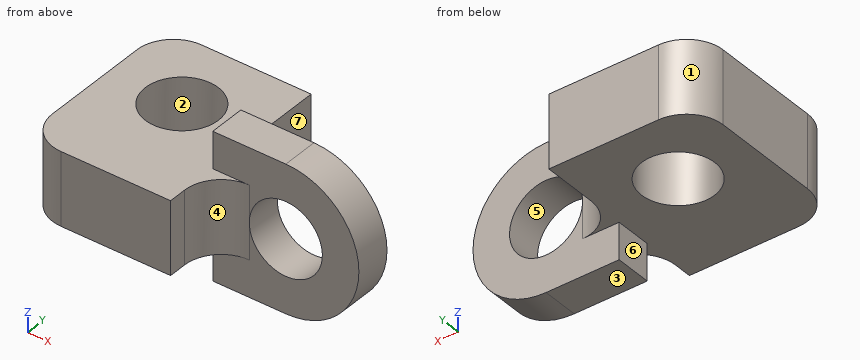
```python
from build123d import *

# Parameters (mm, degrees)
SKETCH_1_R      = 5
EXTRUDE_1_DEPTH = 2.5
SKETCH_2_R      = 5
EXTRUDE_2_DEPTH = 5
FILLET_1_R      = 5
SCALE_1_SCALE   = 0.2


with BuildPart() as part:
    # 草圖1 → 填料-伸長1 (new, symmetric)
    with BuildSketch(Plane(origin=(0, 0, 0), x_dir=(1, 0, 0), z_dir=(0, 1, 0))):
        with BuildLine():
            Line((0, 10), (-10, 10))
            Line((-10, 10), (-10, -10))
            Line((-10, -10), (0, -10))
            ThreePointArc((0, -10), (10, 0), (0, 10))
        make_face()
        with Locations(Location((0, 0, 0), (0, 0, 270))):
            Circle(SKETCH_1_R, mode=Mode.SUBTRACT)
    extrude(amount=EXTRUDE_1_DEPTH, both=True)

    # 草圖2 → 填料-伸長2 (add, symmetric)
    with BuildSketch(Plane.XY):
        with BuildLine():
            Line((-30, 1.898257061), (-30, -5))
            ThreePointArc((-30, -5), (-28.535533906, -8.535533906), (-25, -10))
            Line((-25, -10), (-10, -10))
            Line((-10, -10), (-10, -2.5))
            Line((-10, -2.5), (-10, 2.5))
            Line((-10, 2.5), (-10, 15))
            Line((-10, 15), (-25, 15))
            ThreePointArc((-25, 15), (-28.535533906, 13.535533906), (-30, 10))
            Line((-30, 10), (-30, 1.898257061))
        make_face()
        with Locations((-20, 5)):
            Circle(SKETCH_2_R, mode=Mode.SUBTRACT)
    extrude(amount=EXTRUDE_2_DEPTH, both=True)

    # 圓角1
    fillet_1_edges = [part.edges().sort_by_distance(p)[0] for p in [
        (-10, -2.5, 0),
        (-10, 2.5, 0),
    ]]
    fillet(fillet_1_edges, radius=FILLET_1_R)


with BuildPart() as part_1:
    # 縮放比例1: scaled about (-14.947063882, 1.481061389, 0)
    add(part.part.scale(SCALE_1_SCALE).moved(Location((-11.957651106, 1.184849111, 0))))


solid = part_1.part
```
Geometry check sheet. Reference: the model listing, model coordinates, mm. Face numbers are marked on the shaded views. A direction names the side the tool comes from. Give positions to 0.01 mm unless a question says otherwise; leave off trailing zeros. Write each loop counter-clockwise with the first axis right and the second up, starting at its lowest first coordinate (ties: lowest second). Pieces come first, ordered by that corner, then holes.
1) Release check for a two-part mould opening along X. For the marked faces 1, 2, 3 and 4 record: pulls with the +X half, pulls with the -X half, needs draft (parallel to the pull), parting line crosses it, or undercut.
2) Access from +Z, -Z, +X, -X, +Y, -Y to the whole of each face (thin tool, end or side, straight path). Record for the marked faces 5, 6 and 7.
3) Material ranges on L1, parallel to X at y = 1.15, z = 0; L2, parallel to Y at x = -13.25, z = -1.55; L3, parallel to X at y = 2.3, z = -0.45, recorded low to high.
4) Section check B-B, the plane z = 0.8. Record the boundary of the cut face in (x, y).
5) Gauge pin test, flat ends, axial feed: pin 1 (0.5 mm diameter, centred on y = 1, z = -1.5, fed in from -X); pin 2 (1.5 mm diameter, centred on x = -13, z = 0.5, fed in from +Y); pin 3 (1.2 mm diameter, centred on x = -12.5, z = -1, fed in from -Y). Record the tip position at first contact, or that the pin passes through.
6) Section check C-C, the plane z = 1.6. Record the boundary of the cut face in (x, y).
7) Section check D-D, the plane z = -1.7. Record the boundary of the cut face in (x, y), and give its area (3 significant figures).
8) Section check A-A, the plane y = 0.85. Record the boundary of the cut face in (x, z).
Computed:
1. face 1: pulls with the -X half
1. face 2: undercut
1. face 3: needs draft
1. face 4: pulls with the +X half
2. face 5: +Y, -Y
2. face 6: -Z, -X, +Y, -Y
2. face 7: +Z, -Z, +X, +Y
3. L1: x = -17.96 to -12.96, -10.96 to -9.96
3. L2: y = 0.68 to 1.68
3. L3: x = -17.96 to -16.95, -14.96 to -13.88
4. outline: (-17.96, 0.18) arc R1 ccw to (-16.96, -0.82) - (-13.96, -0.82) - (-13.96, -0.32) arc R1 cw to (-12.96, 0.68) - (-12.56, 0.68) - (-12.56, 1.68) - (-12.96, 1.68) arc R1 cw to (-13.96, 2.68) - (-13.96, 4.18) - (-16.96, 4.18) arc R1 ccw to (-17.96, 3.18) - close; (-11.36, 0.68) - (-10.12, 0.68) - (-10.12, 1.68) - (-11.36, 1.68) - close; hole circle Ø2 at (-15.96, 2.18)
5. pin 1: stops at x = -13.96
5. pin 2: stops at y = 2.07
5. pin 3: stops at y = 0.67
6. outline: (-13.96, 0.68) - (-10.76, 0.68) - (-10.76, 1.68) - (-13.96, 1.68) - close
7. outline: (-13.96, 0.68) - (-10.9, 0.68) - (-10.9, 1.68) - (-13.96, 1.68) - close
7. area: 3.05 mm2
8. outline: (-17.96, -1) - (-13.96, -1) - (-13.96, -2) - (-11.96, -2) arc R2 ccw to (-11.96, 2) - (-13.96, 2) - (-13.96, 1) - (-17.96, 1) - close; hole circle Ø2 at (-11.96, 0)
